```python
from build123d import *

# Parameters (mm, degrees)
SKETCH1_R           = 2.5
BOSS_EXTRUDE1_DEPTH = 10
CUT_EXTRUDE2_DEPTH  = 12


with BuildPart() as part:
    # Sketch1 → Boss-Extrude1 (new body)
    with BuildSketch(Plane.XY):
        Circle(SKETCH1_R)
    extrude(amount=BOSS_EXTRUDE1_DEPTH)

    # Sketch5 → Cut-Extrude2 (cut)
    with BuildSketch(Plane(origin=(0, -3.454207271, 10.011855364), x_dir=(1, 0, 0), z_dir=(0, -0.3396060060418324, 0.9405677863186231))):
        with BuildLine():
            Line((0, 0), (-1.926383071, 1.746152417))
            ThreePointArc((-1.926383071, 1.746152417), (0, -2.6), (1.926383071, 1.746152417))
            Line((1.926383071, 1.746152417), (0, 0))
        make_face()
    extrude(amount=-CUT_EXTRUDE2_DEPTH, mode=Mode.SUBTRACT)


solid = part.part
```
Work out the finished part from the listing and answer in its coordinate system (mm). A direction names the side the tool comes from. Round coordinates to 2 decimals unless told otherwise and drop trailing zeros. Write each loop counter-clockwise with the first axis right and the second up, starting at its lowest first coordinate (ties: lowest second). Pieces come first, ordered by that corner, then holes. Notation, with made-up numbers: (25, 82.25) -> (33, 82.25) arc R22 ccw to (33, 110.25) -> close; hole circle Ø1 at (-27.75, -14.5). An arc over 180 degrees is marked (long way). Write each question's results on one line, items separated by ' | '.
Q1. Determine the mould class of faces 1 (the cylindrical face through (0.1, 2.5, 6)), 2 (the flat face through (0, 2, 0)), 3 (the cylindrical face through (-2.201, -0.009, 4.545)) for opening direction X: released by +X, released by -X, zero draft, split by the parting line, or undercut.
Data:
face 1: split by the parting line | face 2: zero draft | face 3: undercut
Q2. Section A-A, the plane x = -0.95 is taken. Write down the section's boundary in (y, z).
Data:
outline: (-2.31, 9.39) -> (1.08, 0) -> (2.31, 0) -> (2.31, 10) -> (-2.31, 10) -> close
Q3. Which of the six approach directions +Z, -Z, +X, -X, +Y, -Y give full straight-line access (tool end or side, diameter ignored) to faces 4 (the flat face through (0.977, -0.657, 4.873)), 5 (the flat face through (0, 0, 10))?
Data:
face 4: -Z, -Y | face 5: +Z, +X, -X, +Y, -Y
Q4. Flat-ended cylindrical pins translate along their axes: P1, Ø1, axis at x = -2, z = 7, coming from the +Y side; P2, Ø1, axis at x = 1, z = 8.5, coming from the +Y side; P3, Ø1.5, axis at y = 1.5, z = 8, coming from the -X side. Find the tip coordinate at first contact, or state that the pin passes through.
Data:
P1: y = 2 | P2: y = 2.45 | P3: x = -2.38
Q5. Straight lines are drawn through the part: line 1 along X through (y, z) = (1.7, 7.25); line 2 along Y through (x, z) = (-0.3, 7.5); line 3 along Y through (x, z) = (-1.7, 3). For each, find the intervals that lie inside material, in ascending order. Write a range as [from, to].
Data:
line 1: [-1.83, 1.83] | line 2: [-2.26, 2.48] | line 3: [0.72, 1.83]
